from build123d import *

# Parameters (mm, degrees)
SKETCH4_R           = 3.175
SKETCH4_R_2         = 3.25
BOSS_EXTRUDE1_DEPTH = 2.54
SKETCH5_R           = 12.7
CUT_EXTRUDE1_DEPTH  = 5.08
BOSS_EXTRUDE2_DEPTH = 2.54


with BuildPart() as part:
    # Sketch4 → Boss-Extrude1 (new body)
    with BuildSketch(Plane.XY):
        with BuildLine():
            Line((-176.74227619, 45.132498501), (-186.294911373, 53.501319271))
            Line((-186.294911373, 53.501319271), (-184.20270618, 55.889478066))
            Line((-184.20270618, 55.889478066), (-99.572707218, 93.889403295))
            ThreePointArc((-99.572707218, 93.889403295), (-95.936400091, 96.645129164), (-93.872658654, 100.714247725))
            Line((-93.872658654, 100.714247725), (-73.734272023, 181.984262474))
            Line((-73.734272023, 181.984262474), (-71.64206683, 184.372421269))
            Line((-71.64206683, 184.372421269), (-58.940232346, 173.244667072))
            ThreePointArc((-58.940232346, 173.244667072), (17.165554399, 98.128149473), (101.640161914, 32.564267056))
            Line((101.640161914, 32.564267056), (114.125157675, 21.626479751))
            Line((114.125157675, 21.626479751), (112.032952483, 19.238320955))
            Line((112.032952483, 19.238320955), (34.250907029, -11.547413739))
            ThreePointArc((34.250907029, -11.547413739), (30.507681387, -14.12116226), (28.260245615, -18.068940382))
            Line((28.260245615, -18.068940382), (1.564518325, -106.856463453))
            Line((1.564518325, -106.856463453), (-0.527686867, -109.244622248))
            Line((-0.527686867, -109.244622248), (-10.080322049, -100.875801479))
            ThreePointArc((-10.080322049, -100.875801479), (-80.021168146, -12.587414945), (-176.74227619, 45.132498501))
        make_face()
        with Locations((-160.278926398, 53.978352412)):
            Circle(SKETCH4_R, mode=Mode.SUBTRACT)
        with Locations((-3.529256732, -83.108546775)):
            Circle(SKETCH4_R, mode=Mode.SUBTRACT)
        with Locations((81.919540542, 22.826625413)):
            Circle(SKETCH4_R, mode=Mode.SUBTRACT)
        with Locations((-65.999265009, 152.414529532)):
            Circle(SKETCH4_R, mode=Mode.SUBTRACT)
        with Locations((-95.775994763, 64.547904473)):
            Circle(SKETCH4_R_2, mode=Mode.SUBTRACT)
        with Locations((-92.345604955, 12.616132759)):
            Circle(SKETCH4_R_2, mode=Mode.SUBTRACT)
        with Locations((-53.198645122, -21.679523284)):
            Circle(SKETCH4_R_2, mode=Mode.SUBTRACT)
        with Locations((-1.266873408, -18.249133476)):
            Circle(SKETCH4_R_2, mode=Mode.SUBTRACT)
        with Locations((33.028782635, 20.897826357)):
            Circle(SKETCH4_R_2, mode=Mode.SUBTRACT)
        with Locations((29.598392827, 72.829598071)):
            Circle(SKETCH4_R_2, mode=Mode.SUBTRACT)
        with Locations((-9.548567006, 107.125254114)):
            Circle(SKETCH4_R_2, mode=Mode.SUBTRACT)
        with Locations((-61.48033872, 103.694864306)):
            Circle(SKETCH4_R_2, mode=Mode.SUBTRACT)
        with BuildLine():
            Line((-83.124086465, 108.558482428), (-72.906170409, 144.859339501))
            ThreePointArc((-72.906170409, 144.859339501), (-71.703410878, 146.386634264), (-69.772970974, 146.616115326))
            Line((-69.772970974, 146.616115326), (-67.788615701, 146.057561693))
            ThreePointArc((-67.788615701, 146.057561693), (-64.531511448, 145.975700797), (-61.631660764, 147.461061135))
            Line((-61.631660764, 147.461061135), (-53.995233146, 154.194301567))
            ThreePointArc((-53.995233146, 154.194301567), (-52.156051315, 154.824118981), (-50.410205207, 153.968969201))
            Line((-50.410205207, 153.968969201), (-25.527970385, 125.74906719))
            ThreePointArc((-25.527970385, 125.74906719), (-24.735411209, 120.240061903), (-29.468069359, 117.311028592))
            ThreePointArc((-29.468069359, 117.311028592), (-53.532229742, 113.969062176), (-75.246987371, 103.073106251))
            ThreePointArc((-75.246987371, 103.073106251), (-81.13713529, 103.013263889), (-83.124086465, 108.558482428))
        make_face(mode=Mode.SUBTRACT)
        with BuildLine():
            Line((16.986640929, -25.648722449), (3.285829101, -66.077745579))
            ThreePointArc((3.285829101, -66.077745579), (-6.63716699, -74.525917572), (-18.776818461, -69.786052217))
            Line((-18.776818461, -69.786052217), (-42.034504369, -39.805719002))
            ThreePointArc((-42.034504369, -39.805719002), (-42.485464898, -34.268691956), (-37.596964591, -31.62963935))
            ThreePointArc((-37.596964591, -31.62963935), (-13.10838548, -29.619424245), (9.399371164, -19.763849047))
            ThreePointArc((9.399371164, -19.763849047), (15.288833977, -20.004169525), (16.986640929, -25.648722449))
        make_face(mode=Mode.SUBTRACT)
        with BuildLine():
            Line((40.69710548, 0.081884812), (75.33851288, 14.985942183))
            ThreePointArc((75.33851288, 14.985942183), (76.694329343, 16.379147659), (76.667891318, 18.322999714))
            Line((76.667891318, 18.322999714), (75.853173782, 20.216642591))
            ThreePointArc((75.853173782, 20.216642591), (75.343592919, 23.434678742), (76.434608248, 26.504713738))
            Line((76.434608248, 26.504713738), (82.104868563, 34.960463346))
            ThreePointArc((82.104868563, 34.960463346), (82.487292302, 36.86650948), (81.409928575, 38.484702046))
            Line((81.409928575, 38.484702046), (50.16227754, 59.438765709))
            ThreePointArc((50.16227754, 59.438765709), (44.596887673, 59.499797903), (42.315826006, 54.422983254))
            ThreePointArc((42.315826006, 54.422983254), (42.168235941, 30.128317757), (34.223256987, 7.169008885))
            ThreePointArc((34.223256987, 7.169008885), (34.938709714, 1.322167772), (40.69710548, 0.081884812))
        make_face(mode=Mode.SUBTRACT)
        with BuildLine():
            Line((-105.512311204, 81.669494492), (-143.713248966, 62.806648573))
            ThreePointArc((-143.713248966, 62.806648573), (-150.782631627, 51.862619993), (-144.494183598, 40.451951557))
            Line((-144.494183598, 40.451951557), (-111.798776698, 21.36105828))
            ThreePointArc((-111.798776698, 21.36105828), (-106.250665651, 21.63862745), (-104.273833103, 26.83003515))
            ThreePointArc((-104.273833103, 26.83003515), (-105.486548337, 51.342432917), (-98.680560053, 74.92223033))
            ThreePointArc((-98.680560053, 74.92223033), (-99.693477447, 80.728909632), (-105.512311204, 81.669494492))
        make_face(mode=Mode.SUBTRACT)
        with BuildLine():
            Line((93.329108368, 30.491933184), (94.570600217, 29.65941303))
            ThreePointArc((94.570600217, 29.65941303), (96.24244212, 26.144229017), (93.954385503, 22.995202038))
            Line((93.954385503, 22.995202038), (91.863858259, 22.095777322))
            ThreePointArc((91.863858259, 22.095777322), (90.11439141, 22.0719831), (88.860506481, 23.292217917))
            Line((88.860506481, 23.292217917), (88.136116535, 24.97591294))
            ThreePointArc((88.136116535, 24.97591294), (87.959723159, 26.089848531), (88.337382312, 27.152552952))
            Line((88.337382312, 27.152552952), (90.157293538, 29.866487195))
            ThreePointArc((90.157293538, 29.866487195), (91.613666847, 30.83611455), (93.329108368, 30.491933184))
        make_face(mode=Mode.SUBTRACT)
        with BuildLine():
            Line((-60.104144331, 161.506711917), (-62.555111231, 159.345629503))
            ThreePointArc((-62.555111231, 159.345629503), (-63.558905699, 158.831466309), (-64.686364863, 158.859802773))
            Line((-64.686364863, 158.859802773), (-66.450715015, 159.356429663))
            ThreePointArc((-66.450715015, 159.356429663), (-67.825280301, 160.438913241), (-68.031813258, 162.176309155))
            Line((-68.031813258, 162.176309155), (-67.41518612, 164.366980273))
            ThreePointArc((-67.41518612, 164.366980273), (-64.594485575, 167.049371452), (-60.889934446, 165.854434246))
            Line((-60.889934446, 165.854434246), (-59.901345202, 164.733237062))
            ThreePointArc((-59.901345202, 164.733237062), (-59.334509529, 163.077973415), (-60.104144331, 161.506711917))
        make_face(mode=Mode.SUBTRACT)
        with BuildLine():
            ThreePointArc((-58.363398568, 97.382472993), (-71.543951219, -3.129778676), (26.361239359, 23.157354329))
            ThreePointArc((26.361239359, 23.157354329), (8.796739091, 88.575509506), (-58.363398568, 97.382472993))
        make_face(mode=Mode.SUBTRACT)
    extrude(amount=BOSS_EXTRUDE1_DEPTH)

    # Sketch5 → Cut-Extrude1 (cut)
    with BuildSketch(Plane.XY):
        with Locations((-71.64206683, 184.372421269)):
            Circle(SKETCH5_R)
        with Locations((-186.294911373, 53.501319271)):
            Circle(SKETCH5_R)
        with Locations((-0.527686867, -109.244622248)):
            Circle(SKETCH5_R)
        with Locations((114.125157675, 21.626479751)):
            Circle(SKETCH5_R)
    extrude(amount=CUT_EXTRUDE1_DEPTH, mode=Mode.SUBTRACT)

    # Sketch4_4 → Boss-Extrude2 (add)
    with BuildSketch(Plane.XY):
        with BuildLine():
            Line((93.954385503, 22.995202038), (91.863858259, 22.095777322))
            ThreePointArc((91.863858259, 22.095777322), (90.11439141, 22.0719831), (88.860506481, 23.292217917))
            Line((88.860506481, 23.292217917), (88.136116535, 24.97591294))
            ThreePointArc((88.136116535, 24.97591294), (87.959723159, 26.089848531), (88.337382312, 27.152552952))
            Line((88.337382312, 27.152552952), (90.157293538, 29.866487195))
            ThreePointArc((90.157293538, 29.866487195), (91.613666847, 30.83611455), (93.329108368, 30.491933184))
            Line((93.329108368, 30.491933184), (94.570600217, 29.65941303))
            ThreePointArc((94.570600217, 29.65941303), (96.24244212, 26.144229017), (93.954385503, 22.995202038))
        make_face()
        with BuildLine():
            ThreePointArc((-67.41518612, 164.366980273), (-64.594485575, 167.049371452), (-60.889934446, 165.854434246))
            Line((-60.889934446, 165.854434246), (-59.901345202, 164.733237062))
            ThreePointArc((-59.901345202, 164.733237062), (-59.334509529, 163.077973415), (-60.104144331, 161.506711917))
            Line((-60.104144331, 161.506711917), (-62.555111231, 159.345629503))
            ThreePointArc((-62.555111231, 159.345629503), (-63.558905699, 158.831466309), (-64.686364863, 158.859802773))
            Line((-64.686364863, 158.859802773), (-66.450715015, 159.356429663))
            ThreePointArc((-66.450715015, 159.356429663), (-67.825280301, 160.438913241), (-68.031813258, 162.176309155))
            Line((-68.031813258, 162.176309155), (-67.41518612, 164.366980273))
        make_face()
    extrude(amount=BOSS_EXTRUDE2_DEPTH)


solid = part.part
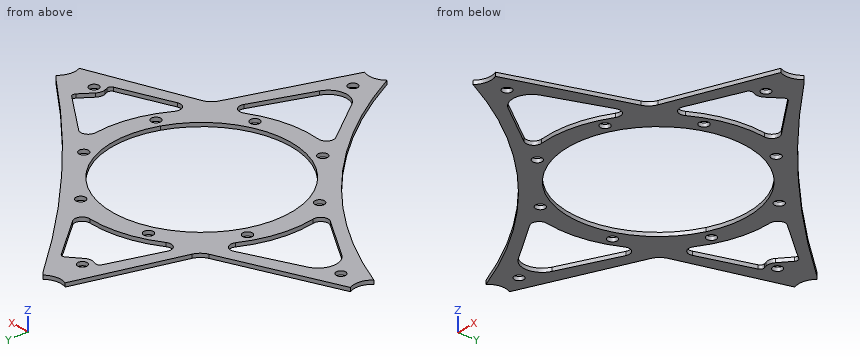
The model under review builds one solid part; all positions refer to its coordinate system, in mm. Round coordinates to 2 decimals unless told otherwise and drop trailing zeros. Write each loop counter-clockwise with the first axis right and the second up, starting at its lowest first coordinate (ties: lowest second). Pieces come first, ordered by that corner, then holes. Notation, with made-up numbers: (-17, 89.5) -> (5, 89.5) arc R18 cw to (5, 112.5) -> close; hole circle Ø6 at (56, 60). An arc over 180 degrees is marked (long way). Answer as a JSON object with one key per item and string values.
1. We need section A-A on x = -133.5. State the section outline as (y, z) points, and give its area (3 significant figures).
Results found:
{"outline": "(25.14, 0) -> (34.03, 0) -> (34.03, 2.54) -> (25.14, 2.54) -> close; (67.85, 0) -> (78.66, 0) -> (78.66, 2.54) -> (67.85, 2.54) -> close", "area": "50.0 mm^2"}
2. To check wall thickness, follow line 1 along X through (y, z) = (64, 2.2); line 2 along Y through (x, z) = (-27.5, 1.8); line 3 along Y through (x, z) = (-21, 2.2). State the ranges of each line that lie inside material, in increasing order.
Results found:
{"line 1": "x = -166.14 to -141.3, -102.89 to -98.98, -92.57 to -88.5, 25.75 to 58.55", "line 2": "y = -71.99 to -58.54, -31.79 to -18.11, 103.56 to 117.65, 127.99 to 140.03", "line 3": "y = -81.96 to -66.92, -31.16 to -17.35, 102.79 to 133.57"}
3. We need section C-C on z = 1.4. State how many separate pieces and enclosed holes the cut face has, and give its area (3 significant figures).
Results found:
{"separate pieces": "1", "enclosed holes": "17", "area": "12,600 mm^2"}
4. We need section B-B on y = -36. State the section outline as (x, z) points.
Results found:
{"outline": "(-56.03, 0) -> (-43.05, 0) -> (-43.05, 2.54) -> (-56.03, 2.54) -> close; (13.48, 0) -> (22.87, 0) -> (22.87, 2.54) -> (13.48, 2.54) -> close"}
5. Clearance check with flat-ended pins moving along their axes: pin 1 (5 mm diameter, centred on x = -66, y = 152.41, fed in from -Z); pin 2 (1 mm diameter, centred on y = 27, z = 2, fed in from +X) (3 decimals). State where each tip first meets the part, or that it passes through.
Results found:
{"pin 1": "passes through", "pin 2": "stops at x = 102.865"}
